The model under review builds one solid part; all positions refer to its coordinate system, in mm. Coordinates: 2 decimals unless noted, no trailing zeros. Loops run counter-clockwise (first coordinate to the right, second up) from the corner with the lowest first, then second, coordinate; pieces in that order, holes last. Notation, with made-up numbers: (23.5, 41.25) - (52.5, 41.25) arc R22 ccw to (52.5, 75.25) - close; hole circle Ø6 at (83.5, 22). An arc over 180 degrees is marked (long way). Use a Markdown table: item, result. Add a question column.
1) Add section B-B, the plane z = 0.75. Give the boundary of the cut face in (x, y), and give its area (3 significant figures).
2) To check wall thickness, follow L1, parallel to Z at x = -3.75, y = 1.75; L2, parallel to Y at x = -3.5, z = 0.05; L3, parallel to Y at x = -1.5, z = -0.05. State the ranges of each line that lie inside material, in increasing order. Write a range as [from, to].
3) Clearance check with a flat-ended pin moving along its axis: pin 1 (2 mm diameter, centred on x = -5.5, y = -0.5, fed in from +Z). State where the tip first meets the part, or that it passes through.
4) Add section A-A, the plane x = 0.5. Give the boundary of the cut face in (y, z).
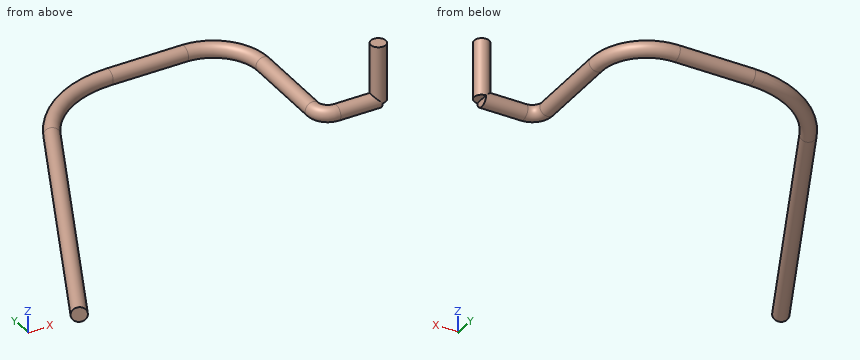
```python
from build123d import *

# Parameters (mm, degrees)
F0_R = 0.15
F6_R = 0.15


with BuildPart() as f2:
    # F2: sweep along a path in F1
    with BuildLine(Plane.XY) as f2_path:
        Line((0, 0), (0, 1.0845226934))
        ThreePointArc((0, 1.0845226934), (-0.2928932188, 1.7916294746), (-1, 2.0845226934))
        Line((-1, 2.0845226934), (-2.505036419, 2.0845226934))
        ThreePointArc((-2.505036419, 2.0845226934), (-3.5683457273, 1.7784451577), (-4.3061999428, 0.9538960083))
        Line((-4.3061999428, 0.9538960083), (-6.8471138366, -4.3103573844))
    # F0 (on Front) → F2 (sweep)
    with BuildSketch(Plane.XZ):
        Circle(F0_R)
    sweep(path=f2_path.line)

    # F4: sweep along a path in F3
    with BuildLine(Plane.XY) as f4_path:
        Line((0, 0), (0, -0.5958363181))
        ThreePointArc((0, -0.5958363181), (0.0878679656, -0.8079683525), (0.3, -0.8958363181))
        Line((0.3, -0.8958363181), (1.136880412, -0.8958363181))
    # F0 (on Front) → F4 (sweep)
    with BuildSketch(Plane.XZ):
        Circle(F0_R)
    sweep(path=f4_path.line)

    # F7: sweep along a path in F5
    with BuildLine(Plane.YZ.offset(1.136880412)) as f7_path:
        Line((-0.8958363181, 0), (-0.8958363181, 1.1528083123))
    # F6 (on Top) → F7 (sweep)
    with BuildSketch(Plane.XY):
        with Locations((1.136880412, -0.8958363181)):
            Circle(F6_R)
    sweep(path=f7_path.line)


solid = f2.part
```
From the geometry:
| question | item | result |
|---|---|---|
| 1 | outline | circle Ø0.3 at (1.14, -0.9) |
| 1 | area | 0.0707 mm^2 |
| 2 | L1 | z = [-0.13, 0.13] |
| 2 | L2 | y = [1.65, 1.98] |
| 2 | L3 | y = [1.94, 2.23] |
| 3 | pin 1 | stops at z = 0.15 |
| 4 | outline | circle Ø0.3 at (-0.9, 0) |
